Build history of the part. All positions in model axes, mm. A direction names the side the tool comes from. Coordinates: 2 decimals unless noted, no trailing zeros. Loops run counter-clockwise (first coordinate to the right, second up) from the corner with the lowest first, then second, coordinate; pieces in that order, holes last. Notation, with made-up numbers: M -18,-19 L 0,-19 A8 ccw 0,-13 Z; hole C 53.25,17.5 d4. An arc over 180 degrees is marked long. Write each question's results on one line, items separated by ' | '. Start each with the question number.
from build123d import *

# Parameters (mm, degrees)
SKETCH1_R           = 1.05
BOSS_EXTRUDE1_DEPTH = 16.5
SKETCH2_R           = 2
BOSS_EXTRUDE2_DEPTH = 2.5
FILLET1_R           = 0.4
FILLET2_R           = 1
SKETCH3_W           = 16.37962499
SKETCH3_H           = 16.511817854
BOSS_EXTRUDE3_DEPTH = 1


with BuildPart() as part:
    # Sketch1 → Boss-Extrude1 (new body)
    with BuildSketch(Plane(origin=(0, 0, 0), x_dir=(1, 0, 0), z_dir=(0, 1, 0))):
        Circle(SKETCH1_R)
    extrude(amount=BOSS_EXTRUDE1_DEPTH)

    # Sketch2 → Boss-Extrude2 (add)
    with BuildSketch(Plane(origin=(0, 16.5, 0), x_dir=(1, 0, 0), z_dir=(0, 1, 0))):
        Circle(SKETCH2_R)
    extrude(amount=BOSS_EXTRUDE2_DEPTH)

    # Fillet1
    fillet1_edges = [part.edges().sort_by_distance(p)[0] for p in [
        (-1.05, 0, 0),
    ]]
    fillet(fillet1_edges, radius=FILLET1_R)

    # Fillet2
    fillet2_edges = [part.edges().sort_by_distance(p)[0] for p in [
        (-2, 19, 0),
    ]]
    fillet(fillet2_edges, radius=FILLET2_R)

    # Sketch3 → Boss-Extrude3 (add)
    with BuildSketch(Plane(origin=(0, 19, 0), x_dir=(1, 0, 0), z_dir=(0, 1, 0))):
        Rectangle(SKETCH3_W, SKETCH3_H)
    extrude(amount=BOSS_EXTRUDE3_DEPTH)


solid = part.part
1. Band-saw the part on A-A, the plane z = 4.75. List the corners of the cut face in (x, y).
2. Pin check, flat tips, straight feed: pin 1 (2 mm diameter, centred on x = 0.5, z = -1, fed in from -Y); pin 2 (2 mm diameter, centred on x = -5, z = 2, fed in from -Y); pin 3 (3 mm diameter, centred on x = 1.5, y = 16, fed in from +Z). Stop position of each tip, or through.
3. Wall check: line 1 along Z through (x, y) = (0, 14.75); line 2 along Y through (x, z) = (-4.5, 3); line 3 along Y through (x, z) = (0.5, -1.5). Give the ranges that are in metal, low to high.
4. Band-saw the part on C-C, the plane x = -5.75. List the corners of the cut face in (y, z), plus the area to 3 significant figures.
5. Band-saw the part on D-D, the plane y = 16.75. List the corners of the cut face in (x, z).
6. Band-saw the part on B-B, the plane y = 7.75. List the corners of the cut face in (x, z).
7. Which spindle directions (+Z, -Z, +X, -X, +Y, -Y) get a long thin tool onto all of the face, cutting with end or side? Do faces 1 (the flat face through (8.19, 19.5, 0.1)), 2 (the cylindrical face through (0, 17, 2)). Say none if no direction does.
Checked values:
1) outline: M -8.19,19 L 8.19,19 L 8.19,20 L -8.19,20 Z
2) pin 1: y = 0 | pin 2: y = 19 | pin 3: z = 2
3) line 1: -1.05 to 1.05 | line 2: 19 to 20 | line 3: 16.5 to 18.81, 19 to 20
4) outline: M 19,-8.26 L 20,-8.26 L 20,8.26 L 19,8.26 Z | area: 16.5 mm²
5) outline: C 0,0 d4
6) outline: C 0,0 d2.1
7) face 1: +Z, -Z, +X, +Y, -Y | face 2: -Y
